The listing builds one solid part. Answer for the finished solid, in the listing's coordinates (mm). A direction names the side the tool comes from. Coordinates: 2 decimals unless noted, no trailing zeros. Order: outer loops, then holes, each group sorted by start corner. A loop starts at its lowest first (then second) coordinate and runs counter-clockwise, first axis right, second up.
from build123d import *

# Parameters (mm, degrees)
SKETCH_1_R          = 33.5
SKETCH_1_R_2        = 25
SKETCH_1_W          = 80
SKETCH_1_H          = 20
SKETCH_1_R_3        = 2.1
EXTRUDE_1_DEPTH     = 6
SKETCH_3_R          = 2.05
CUT_EXTRUDE_1_DEPTH = 7
EXTRUDE_2_DEPTH     = 6
FILLET_1_R          = 2
SKETCH_5_W          = 80
SKETCH_5_H          = 3
EXTRUDE_3_DEPTH     = 6
FILLET_2_R          = 5
SKETCH_6_W          = 50
SKETCH_6_H          = 20
CUT_EXTRUDE_2_DEPTH = 10
FILLET_3_R          = 3
FILLET_4_R          = 1.5
FILLET_5_R          = 5
SKETCH_7_R          = 2.025
CUT_EXTRUDE_3_DEPTH = 10


with BuildPart() as part:
    # 草图1 → 凸台-拉伸1 (new body)
    with BuildSketch(Plane.XY):
        with Locations((0, 85.5)):
            Circle(SKETCH_1_R)
        with Locations((0, 85.5)):
            Circle(SKETCH_1_R_2, mode=Mode.SUBTRACT)
        with BuildLine():
            Line((-33.38100662, 88.32106311), (-40, 10))
            Line((-40, 10), (40, 10))
            Line((40, 10), (33.38100662, 88.32106311))
            ThreePointArc((33.38100662, 88.32106311), (33.470238435, 86.911785792), (33.5, 85.5))
            ThreePointArc((33.5, 85.5), (-1.411785792, 52.029761565), (-33.38100662, 88.32106311))
        make_face()
        Rectangle(SKETCH_1_W, SKETCH_1_H)
        with Locations((-30, 7.5)):
            Circle(SKETCH_1_R_3, mode=Mode.SUBTRACT)
        with Locations((30, 7.5)):
            Circle(SKETCH_1_R_3, mode=Mode.SUBTRACT)
        with Locations((30, -7.5)):
            Circle(SKETCH_1_R_3, mode=Mode.SUBTRACT)
        with Locations((-30, -7.5)):
            Circle(SKETCH_1_R_3, mode=Mode.SUBTRACT)
    extrude(amount=EXTRUDE_1_DEPTH)

    # 草图3 → 切除-拉伸1 (cut, through all)
    with BuildSketch(Plane.XY.offset(6)):
        with Locations((0, 114.5)):
            Circle(SKETCH_3_R)
        with Locations((14.5, 110.61473671)):
            Circle(SKETCH_3_R)
        with Locations((25.11473671, 100)):
            Circle(SKETCH_3_R)
        with Locations((29, 85.5)):
            Circle(SKETCH_3_R)
        with Locations((25.11473671, 71)):
            Circle(SKETCH_3_R)
        with Locations((14.5, 60.38526329)):
            Circle(SKETCH_3_R)
        with Locations((0, 56.5)):
            Circle(SKETCH_3_R)
        with Locations((-14.5, 60.38526329)):
            Circle(SKETCH_3_R)
        with Locations((-25.11473671, 71)):
            Circle(SKETCH_3_R)
        with Locations((-29, 85.5)):
            Circle(SKETCH_3_R)
        with Locations((-25.11473671, 100)):
            Circle(SKETCH_3_R)
        with Locations((-14.5, 110.61473671)):
            Circle(SKETCH_3_R)
    extrude(amount=-CUT_EXTRUDE_1_DEPTH, mode=Mode.SUBTRACT)


with BuildPart() as body_2:
    # 草图4 → 凸台-拉伸2 (new body)
    with BuildSketch(Plane.XY.offset(6)):
        with BuildLine():
            ThreePointArc((-10.272279454, 108.292109925), (-12.5, 107.150635095), (-14.602406473, 105.792109925))
            Line((-14.602406473, 105.792109925), (-9.560163238, 97.058688457))
            Line((-9.560163238, 97.058688457), (-7.77754959, 93.971111048))
            ThreePointArc((-7.77754959, 93.971111048), (-5.75, 95.459292144), (-3.447422571, 96.471111048))
            Line((-3.447422571, 96.471111048), (-5.230036219, 99.558688457))
            Line((-5.230036219, 99.558688457), (-10.272279454, 108.292109925))
        make_face()
        with BuildLine():
            ThreePointArc((25, 85.5), (24.968651828, 86.751569376), (24.874685928, 88))
            Line((24.874685928, 88), (14.790199458, 88))
            Line((14.790199458, 88), (11.22497216, 88))
            ThreePointArc((11.22497216, 88), (11.431036258, 86.757541283), (11.5, 85.5))
            ThreePointArc((11.5, 85.5), (11.431036258, 84.242458717), (11.22497216, 83))
            Line((11.22497216, 83), (14.790199458, 83))
            Line((14.790199458, 83), (24.874685928, 83))
            ThreePointArc((24.874685928, 83), (24.968651828, 84.248430624), (25, 85.5))
        make_face()
        with BuildLine():
            Line((-9.560163238, 73.941311543), (-14.602406473, 65.207890075))
            ThreePointArc((-14.602406473, 65.207890075), (-12.5, 63.849364905), (-10.272279454, 62.707890075))
            Line((-10.272279454, 62.707890075), (-5.230036219, 71.441311543))
            Line((-5.230036219, 71.441311543), (-3.447422571, 74.528888952))
            ThreePointArc((-3.447422571, 74.528888952), (-5.75, 75.540707856), (-7.77754959, 77.028888952))
            Line((-7.77754959, 77.028888952), (-9.560163238, 73.941311543))
        make_face()
        with BuildLine():
            Line((-7.77754959, 93.971111048), (-9.560163238, 97.058688457))
            ThreePointArc((-9.560163238, 97.058688457), (-15, 85.5), (-9.560163238, 73.941311543))
            Line((-9.560163238, 73.941311543), (-7.77754959, 77.028888952))
            ThreePointArc((-7.77754959, 77.028888952), (-11.5, 85.5), (-7.77754959, 93.971111048))
        make_face()
        with BuildLine():
            Line((-3.447422571, 74.528888952), (-5.230036219, 71.441311543))
            ThreePointArc((-5.230036219, 71.441311543), (7.5, 72.509618943), (14.790199458, 83))
            Line((14.790199458, 83), (11.22497216, 83))
            ThreePointArc((11.22497216, 83), (5.75, 75.540707856), (-3.447422571, 74.528888952))
        make_face()
        with BuildLine():
            ThreePointArc((14.790199458, 88), (7.5, 98.490381057), (-5.230036219, 99.558688457))
            Line((-5.230036219, 99.558688457), (-3.447422571, 96.471111048))
            ThreePointArc((-3.447422571, 96.471111048), (5.75, 95.459292144), (11.22497216, 88))
            Line((11.22497216, 88), (14.790199458, 88))
        make_face()
    extrude(amount=-EXTRUDE_2_DEPTH)

    # Combine 1: union part
    add(part.part)

    # 圆角1
    fillet_1_edges = [body_2.edges().sort_by_distance(p)[0] for p in [
        (-9.560163238, 73.941311543, 3),
        (-14.602406473, 65.207890075, 3),
        (-10.272279454, 62.707890075, 3),
        (-5.230036219, 71.441311543, 3),
        (14.790199458, 83, 3),
        (24.874685928, 83, 3),
        (24.874685928, 88, 3),
        (14.790199458, 88, 3),
        (-5.230036219, 99.558688457, 3),
        (-10.272279454, 108.292109925, 3),
        (-14.602406473, 105.792109925, 3),
        (-9.560163238, 97.058688457, 3),
    ]]
    fillet(fillet_1_edges, radius=FILLET_1_R)

    # 草图5 → 凸台-拉伸3 (add)
    with BuildSketch(Plane.XY.offset(6)):
        with Locations((0, -11.5)):
            Rectangle(SKETCH_5_W, SKETCH_5_H)
    extrude(amount=-EXTRUDE_3_DEPTH)

    # 圆角2
    fillet_2_edges = [body_2.edges().sort_by_distance(p)[0] for p in [
        (-40, -13, 3),
        (40, -13, 3),
    ]]
    fillet(fillet_2_edges, radius=FILLET_2_R)

    # 草图6 → 切除-拉伸2 (cut)
    with BuildSketch(Plane(origin=(0, 0, 0), x_dir=(-1, 0, 0), z_dir=(0, 0, -1))):
        Polygon((-13.279056191, 18), (-3, 18), (-3, 35.803847577), align=None)
        Polygon((3, 35.803847577), (3, 18), (13.279056191, 18), align=None)
        with Locations((0, 2)):
            Rectangle(SKETCH_6_W, SKETCH_6_H)
        Polygon((-33.302523575, 18), (-20.950767875, 18), (-30.401818232, 52.323395297), align=None)
        with BuildLine():
            Line((-16.167580049, 26.996929919), (-3.922674029, 48.205729281))
            ThreePointArc((-3.922674029, 48.205729281), (-14.860033774, 51.069934705), (-24.446601804, 57.063866996))
            Line((-24.446601804, 57.063866996), (-16.167580049, 26.996929919))
        make_face()
        with BuildLine():
            ThreePointArc((24.446601804, 57.063866996), (14.860033774, 51.069934705), (3.922674029, 48.205729281))
            Line((3.922674029, 48.205729281), (16.167580049, 26.996929919))
            Line((16.167580049, 26.996929919), (24.446601804, 57.063866996))
        make_face()
        Polygon((30.401818232, 52.323395297), (20.950767875, 18), (33.302523575, 18), align=None)
    extrude(amount=-CUT_EXTRUDE_2_DEPTH, mode=Mode.SUBTRACT)

    # 圆角3
    fillet_3_edges = [body_2.edges().sort_by_distance(p)[0] for p in [
        (-25, 12, 3),
        (-25, -8, 3),
        (25, -8, 3),
        (25, 12, 3),
    ]]
    fillet(fillet_3_edges, radius=FILLET_3_R)

    # 圆角4
    fillet_4_edges = [body_2.edges().sort_by_distance(p)[0] for p in [
        (-3, 35.803847577, 3),
        (-13.279056191, 18, 3),
        (-3, 18, 3),
        (3, 35.803847577, 3),
        (3, 18, 3),
        (13.279056191, 18, 3),
        (-24.446601804, 57.063866996, 3),
        (-16.167580049, 26.996929919, 3),
        (-20.950767875, 18, 3),
        (-30.401818232, 52.323395297, 3),
        (-33.302523575, 18, 3),
        (20.950767875, 18, 3),
        (33.302523575, 18, 3),
        (30.401818232, 52.323395297, 3),
        (24.446601804, 57.063866996, 3),
        (16.167580049, 26.996929919, 3),
    ]]
    fillet(fillet_4_edges, radius=FILLET_4_R)

    # 圆角5
    fillet_5_edges = [body_2.edges().sort_by_distance(p)[0] for p in [
        (-3.922674029, 48.205729281, 3),
        (3.922674029, 48.205729281, 3),
    ]]
    fillet(fillet_5_edges, radius=FILLET_5_R)

    # 草图7 → 切除-拉伸3 (cut)
    with BuildSketch(Plane(origin=(0, 0, 0), x_dir=(-1, 0, 0), z_dir=(0, 0, -1))):
        with Locations((-30, 55)):
            Circle(SKETCH_7_R)
        with Locations((30, 55)):
            Circle(SKETCH_7_R)
    extrude(amount=-CUT_EXTRUDE_3_DEPTH, mode=Mode.SUBTRACT)


solid = body_2.part
(1) Find section C-C on y = 48. Determine the outline of the cut face in (x, z).
(2) The mould has two halves that part along X. Classify faces 1 (the flat face through (-1, 54, 0)), 2 (the cylindrical face through (29.783, 45.308, 3.042)), 3 (the flat face through (40, 1, 3)): pulls with the +X half, pulls with the -X half, needs draft (parallel to the pull), parting line crosses it, or undercut.
(3) Find section A-A on x = 0. Determine the outline of the cut face in (y, z).
(4) Find the intervals of material crossed by probe 1 along Y at (x, z) = (-9.5, 4); probe 2 along X at (y, z) = (35, 2.75); probe 3 along Y at (x, z) = (-29, 1.95), in increasing order.
(5) Find section B-B on y = 7.5. Determine the outline of the cut face in (x, z), then the cut area to 3 significant figures.
(6) Find section D-D on z = 1.25. Count the separate pieces of the cut face and the enclosed holes in it, then the cut area to 3 significant figures.
(7) A tool of negligible diameter and unlimited length cuts with its end or side. For faces 4 (the cylindrical face through (-4.14, 31.66, 3.04)), 5 (the cylindrical face through (0.697, 118.993, 2.958)), from which of +Z, -Z, +X, -X, +Y, -Y can it reach the whole face along a straight path? Write none if from no direction.
(8) Given pin 1 Ø1.5 at (x, z) = (25.5, 4.5) entering from +Y; pin 2 Ø2 at (x, z) = (-27.5, 4) entering from +Y, each flat-ended and moving along its own axis, determine where each tip first touches the part or whether it passes through.
Resolved:
1. outline: (-36.79, 0) - (-21.95, 0) - (-21.95, 6) - (-36.79, 6) - close; (-8.03, 0) - (8.03, 0) - (8.03, 6) - (-8.03, 6) - close; (21.95, 0) - (36.79, 0) - (36.79, 6) - (21.95, 6) - close
2. face 1: needs draft
2. face 2: undercut
2. face 3: pulls with the +X half
3. outline: (-13, 0) - (-8, 0) - (-8, 6) - (-13, 6) - close; (12, 0) - (54.45, 0) - (54.45, 6) - (12, 6) - close; (58.55, 0) - (60.5, 0) - (60.5, 6) - (58.55, 6) - close; (70.5, 0) - (74, 0) - (74, 6) - (70.5, 6) - close; (97, 0) - (100.5, 0) - (100.5, 6) - (97, 6) - close; (110.5, 0) - (112.45, 0) - (112.45, 6) - (110.5, 6) - close; (116.55, 0) - (119, 0) - (119, 6) - (116.55, 6) - close
4. probe 1: y = -13 to -8, 12 to 18, 24.55 to 38.55, 49.12 to 79.02, 91.98 to 117.62
4. probe 2: x = -37.89 to -31.87, -25.63 to -18.37, -11.55 to 11.55, 18.37 to 25.63, 31.87 to 37.89
4. probe 3: y = -13 to -9.35, -5.65 to 5.65, 9.35 to 18, 45.18 to 53.24, 56.76 to 83.45, 87.55 to 102.27
5. outline: (-40, 0) - (-32.1, 0) - (-32.1, 6) - (-40, 6) - close; (-27.9, 0) - (-25, 0) - (-25, 6) - (-27.9, 6) - close; (25, 0) - (27.9, 0) - (27.9, 6) - (25, 6) - close; (32.1, 0) - (40, 0) - (40, 6) - (32.1, 6) - close
5. area: 130 mm2
6. separate pieces: 1
6. enclosed holes: 29
6. area: 5,380 mm2
7. face 4: +Z, -Z
7. face 5: +Z, -Z, +Y
8. pin 1: stops at y = 108.08
8. pin 2: stops at y = 105.99
